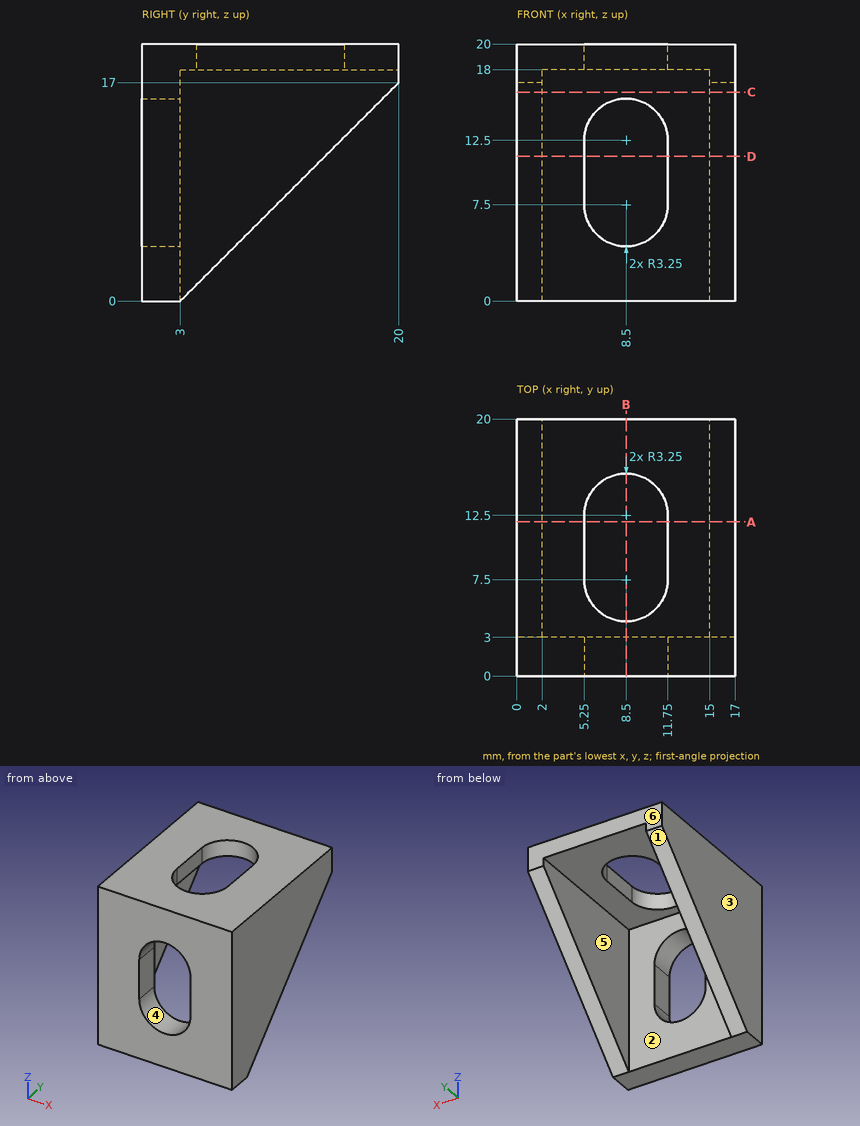
Verification items for this drawing (mm, ordinates from the low corner). A direction names the side the tool comes from. Coordinates: 2 decimals unless noted, no trailing zeros. Loops run counter-clockwise (first coordinate to the right, second up) from the corner with the lowest first, then second, coordinate; pieces in that order, holes last. Notation, with made-up numbers: (53, -27.5) -> (61, -27.5) arc R20 ccw to (61, -14.5) -> close; hole circle Ø6 at (26, -31). An arc over 180 degrees is marked (long way). Answer in a Markdown table with one row per item. Add a question column.
1. Section check C-C, the plane z = 16.25. Enter the section's corners in (x, y), then the cut area to 3 significant figures.
2. Section check A-A, the plane y = 12. Enter the section's corners in (x, z), then the cut area to 3 significant figures.
3. Section check B-B, the plane x = 8.5. Enter the section's corners in (y, z), then the cut area to 3 significant figures.
4. Material ranges on probe 1 along X at (y, z) = (4, 17.5); probe 2 along X at (y, z) = (2, 12.5); probe 3 along Z at (x, y) = (7.5, 19), recorded low to high. Write a range as [from, to].
5. Access from +Z, -Z, +X, -X, +Y, -Y to the whole of each face (thin tool, end or side, straight path). Record for the marked faces 4, 5 and 6.
6. Section check D-D, the plane z = 11.25. Enter the section's corners in (x, y), then the cut area to 3 significant figures.
7. Depth check by flat-ended pin: P1, Ø1.5, axis at x = 10, z = 14, coming from the -Y side; P2, Ø1.5, axis at x = 9.5, y = 18, coming from the -Z side; P3, Ø4, axis at x = 2.5, z = 12.5, coming from the +Y side; P4, Ø10, axis at x = 2.5, y = 17.5, coming from the -Z side. Enter the tip coordinate at first touch or a pass-through.
8. Draft check along X on the marked faces 1, 2 and 3. Enter one of: +X half, -X half, draft (parallel to the pull), parting line (faces both ways), or undercut.
Derived:
| question | item | result |
|---|---|---|
| 1 | outline | (0, 0) -> (17, 0) -> (17, 19.25) -> (15, 19.25) -> (15, 3) -> (2, 3) -> (2, 19.25) -> (0, 19.25) -> close |
| 1 | area | 116 mm² |
| 2 | outline | (0, 9) -> (2, 9) -> (2, 18) -> (5.25, 18) -> (5.25, 20) -> (0, 20) -> close; (11.75, 18) -> (15, 18) -> (15, 9) -> (17, 9) -> (17, 20) -> (11.75, 20) -> close |
| 2 | area | 57.0 mm² |
| 3 | outline | (0, 0) -> (3, 0) -> (3, 4.25) -> (0, 4.25) -> close; (0, 15.75) -> (3, 15.75) -> (3, 18) -> (4.25, 18) -> (4.25, 20) -> (0, 20) -> close; (15.75, 18) -> (20, 18) -> (20, 20) -> (15.75, 20) -> close |
| 3 | area | 36.5 mm² |
| 4 | probe 1 | x = [0, 2], [15, 17] |
| 4 | probe 2 | x = [0, 5.25], [11.75, 17] |
| 4 | probe 3 | z = [18, 20] |
| 5 | face 4 | +Y, -Y |
| 5 | face 5 | -Z, +Y |
| 5 | face 6 | +Z, -Z, +X, -X, +Y |
| 6 | outline | (0, 0) -> (5.25, 0) -> (5.25, 3) -> (2, 3) -> (2, 14.25) -> (0, 14.25) -> close; (11.75, 0) -> (17, 0) -> (17, 14.25) -> (15, 14.25) -> (15, 3) -> (11.75, 3) -> close |
| 6 | area | 76.5 mm² |
| 7 | P1 | passes through |
| 7 | P2 | stops at z = 18 |
| 7 | P3 | stops at y = 17.44 |
| 7 | P4 | stops at z = 9.53 |
| 8 | face 1 | draft |
| 8 | face 2 | undercut |
| 8 | face 3 | -X half |
